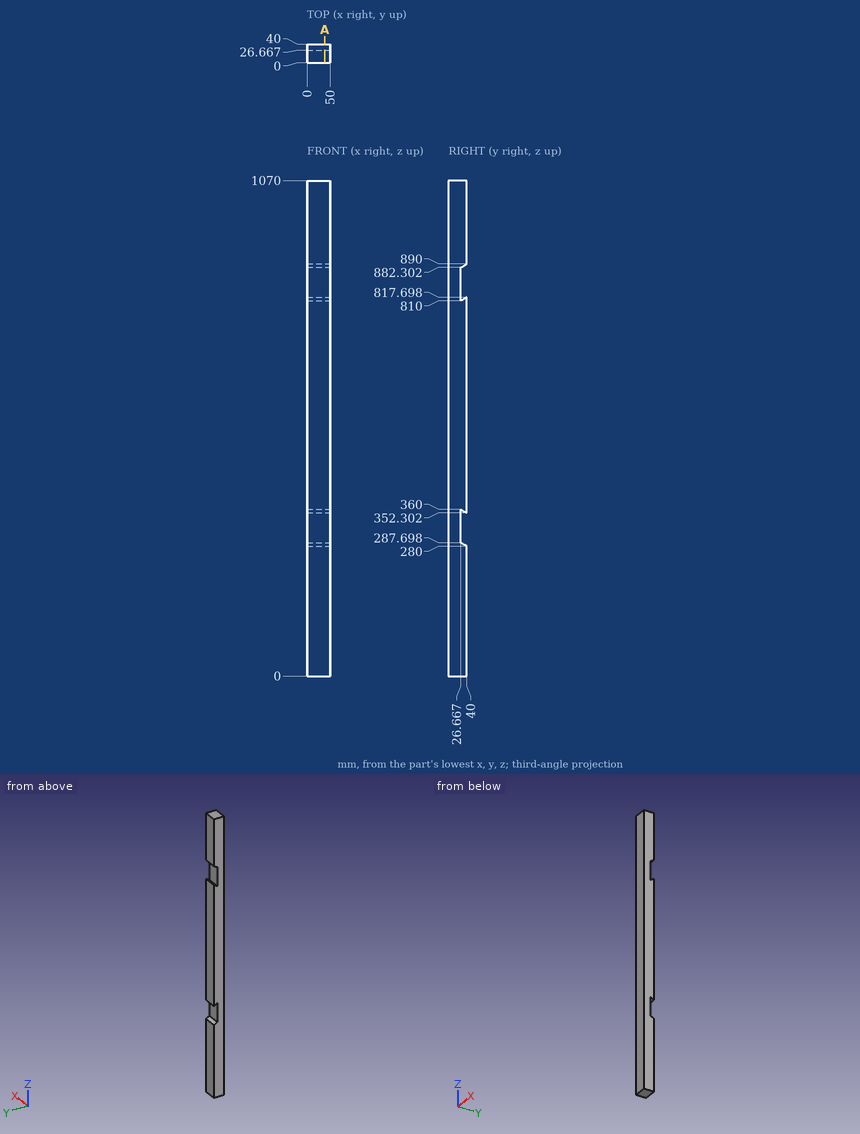
The figure shows three views and two pictorial views of one solid part (mm, origin at its lowest corner). Answer the questions. Round coordinates to 2 decimals unless told otherwise and drop trailing zeros. Order: outer loops, then holes, each group sorted by start corner. A loop starts at its lowest first (then second) coordinate and runs counter-clockwise, first axis right, second up.
Q1. Find the intervals of material crossed by line 1 along Z through (x, y) = (36.5, 35); line 2 along Z through (x, y) = (15.5, 35.5); line 3 along Y through (x, z) = (5.5, 359.5) (1 decimal), in increasing order.
Solution:
line 1: z = 0 to 282.89, 355.19 to 814.81, 887.11 to 1070
line 2: z = 0 to 282.6, 354.9 to 815.1, 887.4 to 1070
line 3: y = 0 to 26.7, 27.5 to 40
Q2. A cutting plane is placed at A-A, the plane x = 38. Determine the outline of the cut face in (y, z).
Solution:
outline: (0, 0) - (40, 0) - (40, 280) - (26.67, 287.7) - (26.67, 360) - (40, 352.3) - (40, 817.7) - (26.67, 810) - (26.67, 882.3) - (40, 890) - (40, 1070) - (0, 1070) - close
Q3. Given pin 1 Ø12 at (y, z) = (28, 689) entering from -X; pin 2 Ø25 at (x, z) = (30.5, 337.5) entering from +Y, each flat-ended and moving along its own axis, determine where each tip first touches the part or whether it passes through.
Solution:
pin 1: stops at x = 0
pin 2: stops at y = 26.67
